Design review of the part shown in the three views and the two pictorial views. Dimensions are in mm from the part's minimum x, y and z. Round coordinates to 2 decimals unless told otherwise and drop trailing zeros. Order: outer loops, then holes, each group sorted by start corner. A loop starts at its lowest first (then second) coordinate and runs counter-clockwise, first axis right, second up. Notation, with made-up numbers: (-38.5, -33) - (11.5, -33) arc R14 ccw to (11.5, -15) - close; hole circle Ø9 at (7.25, -0.5). An arc over 180 degrees is marked (long way). One line per item, written item: value.
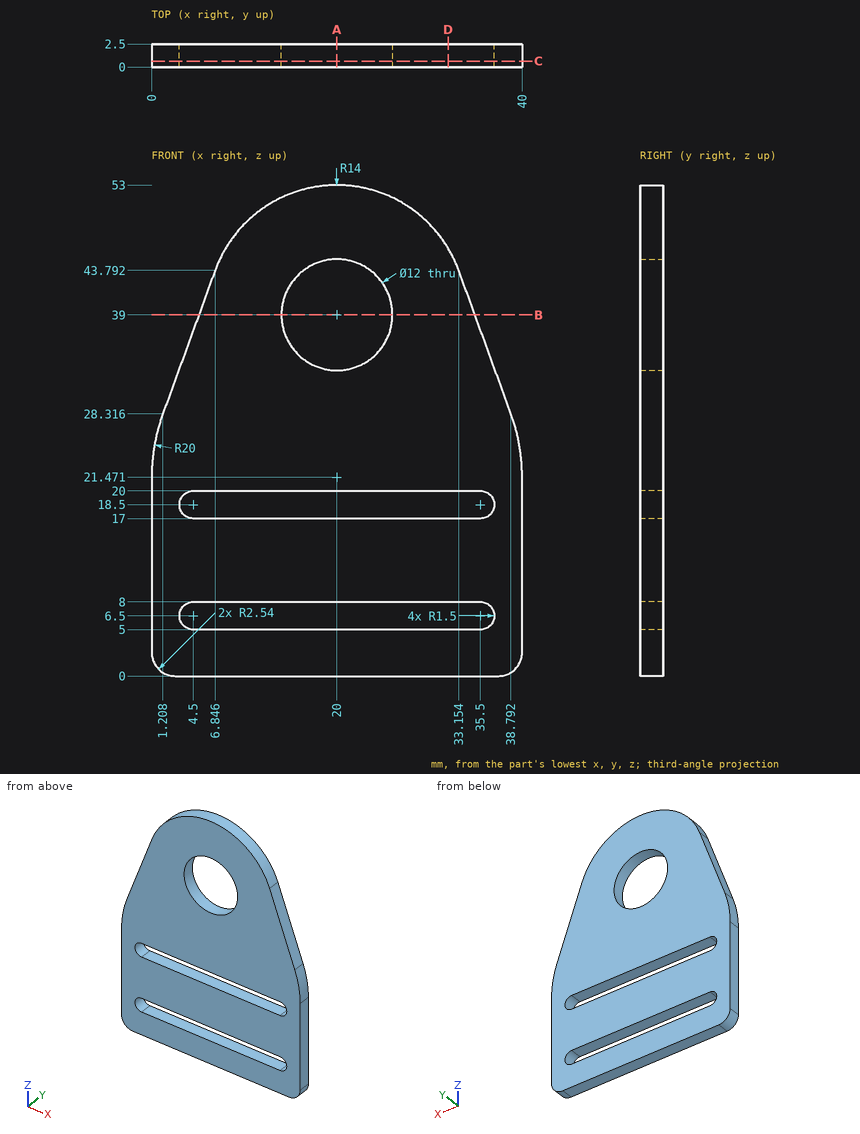
Item 1: Take a section at A-A (x = 20). Write out the cut boundary in (y, z).
Returned:
outline: (0, 0) - (2.5, 0) - (2.5, 5) - (0, 5) - close; (0, 8) - (2.5, 8) - (2.5, 17) - (0, 17) - close; (0, 20) - (2.5, 20) - (2.5, 33) - (0, 33) - close; (0, 45) - (2.5, 45) - (2.5, 53) - (0, 53) - close
Item 2: For P1, Ø9.5, axis at x = 20, z = 39, coming from the +Y side; P2, Ø1.2, axis at x = 15.5, y = 1.5, coming from the +Z side, all flat-tipped, find the tip position at first contact; note any pin that passes through.
Returned:
P1: through
P2: z = 52.45
Item 3: Take a section at B-B (z = 39). Write out the cut boundary in (x, y), plus the area to 3 significant figures.
Returned:
outline: (5.1, 0) - (14, 0) - (14, 2.5) - (5.1, 2.5) - close; (26, 0) - (34.9, 0) - (34.9, 2.5) - (26, 2.5) - close
area: 44.5 mm^2
Item 4: Take a section at C-C (y = 0.65). Write out the cut boundary in (x, z) (1 decimal), plus the area to 3 significant figures.
Returned:
outline: (0, 2.5) arc R2.5 ccw to (2.5, 0) - (37.5, 0) arc R2.5 ccw to (40, 2.5) - (40, 21.5) arc R20 ccw to (38.8, 28.3) - (33.2, 43.8) arc R14 ccw to (6.8, 43.8) - (1.2, 28.3) arc R20 ccw to (0, 21.5) - close; hole (4.5, 5) - (35.5, 5) arc R1.5 ccw to (35.5, 8) - (4.5, 8) arc R1.5 ccw to start; hole (4.5, 17) - (35.5, 17) arc R1.5 ccw to (35.5, 20) - (4.5, 20) arc R1.5 ccw to start; hole circle Ø12 at (20, 39)
area: 1,480 mm^2
Item 5: Wall thickness on line 1 (Z direction, x = 32, y = 1.7); line 2 (Z direction, x = 10, y = 1.25); line 3 (Z direction, x = 17.5, y = 0.55) (1 decimal): over which ranges is each line inside the solid? List them lowest first.
Returned:
line 1: 0 to 5, 8 to 17, 20 to 46.21
line 2: 0 to 5, 8 to 17, 20 to 48.8
line 3: 0 to 5, 8 to 17, 20 to 33.5, 44.5 to 52.8
Item 6: Take a section at D-D (x = 32). Write out the cut boundary in (y, z).
Returned:
outline: (0, 0) - (2.5, 0) - (2.5, 5) - (0, 5) - close; (0, 8) - (2.5, 8) - (2.5, 17) - (0, 17) - close; (0, 20) - (2.5, 20) - (2.5, 46.21) - (0, 46.21) - close
